Could you check a few things on this model? Use its own coordinates, in mm. Round coordinates to 2 decimals unless told otherwise and drop trailing zeros. Write each loop counter-clockwise with the first axis right and the second up, starting at its lowest first coordinate (ties: lowest second). Pieces come first, ordered by that corner, then holes. Notation, with made-up numbers: (62.5, 9) -> (86.5, 9) arc R28 cw to (86.5, 32) -> close; hole circle Ø3 at (24.25, 78.25). An arc over 180 degrees is marked (long way). One line per question, with ' | ' between items. Start each with the question number.
1. Imagine slicing it at B-B, the plane z = 18. List the corners of the cut face in (x, y) for me.
2. Imagine slicing it at A-A, the plane x = 15. List the corners of the cut face in (y, z) for me, and give its area (3 significant figures).
3. Thinking about a two-plate mould opening in Z: for faces 1 (the flat face through (22, 2, 0)), 2 (the flat face through (0, 2, 22)), 3 (the cylindrical face through (13.004, 1.972, 16.038)), 4 (the cylindrical face through (-0.843, 1.972, -15.968)), which applies, released by +Z, released by -Z, zero draft, split by the parting line, or undercut?
4. Imagine slicing it at D-D, the plane x = 0. List the corners of the cut face in (y, z) for me.
5. For pin 1 Ø7 at (x, z) = (0, 18) entering from -Y, with a flat end and sliding along its axis, tell me the tip position at first contact or that it passes through.
6. If I drill on line 1 along X through (y, z) = (1, 15); line 2 along X through (y, z) = (1.8, 18); line 3 along Z through (x, y) = (-2, 3.7), over which ranges is the centre line in solid material (lowest first)? Write a range as [from, to].
7. Imagine slicing it at C-C, the plane y = 1.5. List the corners of the cut face in (x, z) for me.
from build123d import *

# Parameters (mm, degrees)
SK_PLATE_W      = 44
SK_PLATE_H      = 44
EX_PLATE_DEPTH  = 4
SK_HOLES_R      = 2.25
SK_HOLES_R_2    = 2.2
CUT_HOLES_DEPTH = 4


with BuildPart() as part:
    # SK_Plate → EX_Plate (new body)
    with BuildSketch(Plane(origin=(0, 0, 0), x_dir=(1, 0, 0), z_dir=(0, 1, 0))):
        Rectangle(SK_PLATE_W, SK_PLATE_H)
    extrude(amount=EX_PLATE_DEPTH)

    # SK_Holes → CUT_Holes (cut)
    with BuildSketch(Plane(origin=(0, 0, 0), x_dir=(1, 0, 0), z_dir=(0, 1, 0))):
        with Locations(Location((15, -15, 0), (0, 0, 270))):
            Circle(SK_HOLES_R)
        with Locations(Location((-15, -15, 0), (0, 0, 270))):
            Circle(SK_HOLES_R)
        with Locations(Location((15, 15, 0), (0, 0, 270))):
            Circle(SK_HOLES_R)
        with Locations(Location((-15, 15, 0), (0, 0, 270))):
            Circle(SK_HOLES_R)
        with Locations(Location((0, -18, 0), (0, 0, 270))):
            Circle(SK_HOLES_R_2)
        with Locations(Location((0, 18, 0), (0, 0, 270))):
            Circle(SK_HOLES_R_2)
    extrude(amount=CUT_HOLES_DEPTH, mode=Mode.SUBTRACT)


solid = part.part
Geometry results:
1) outline: (-22, 0) -> (-2.2, 0) -> (-2.2, 4) -> (-22, 4) -> close; (2.2, 0) -> (22, 0) -> (22, 4) -> (2.2, 4) -> close
2) outline: (0, -22) -> (4, -22) -> (4, -17.25) -> (0, -17.25) -> close; (0, -12.75) -> (4, -12.75) -> (4, 12.75) -> (0, 12.75) -> close; (0, 17.25) -> (4, 17.25) -> (4, 22) -> (0, 22) -> close | area: 140 mm2
3) face 1: zero draft | face 2: released by +Z | face 3: undercut | face 4: undercut
4) outline: (0, -22) -> (4, -22) -> (4, -20.2) -> (0, -20.2) -> close; (0, -15.8) -> (4, -15.8) -> (4, 15.8) -> (0, 15.8) -> close; (0, 20.2) -> (4, 20.2) -> (4, 22) -> (0, 22) -> close
5) pin 1: stops at y = 0
6) line 1: x = [-22, -17.25], [-12.75, 12.75], [17.25, 22] | line 2: x = [-22, -2.2], [2.2, 22] | line 3: z = [-22, -18.92], [-17.08, 17.08], [18.92, 22]
7) outline: (-22, -22) -> (22, -22) -> (22, 22) -> (-22, 22) -> close; hole circle Ø4.5 at (-15, -15); hole circle Ø4.5 at (-15, 15); hole circle Ø4.4 at (0, -18); hole circle Ø4.4 at (0, 18); hole circle Ø4.5 at (15, -15); hole circle Ø4.5 at (15, 15)
